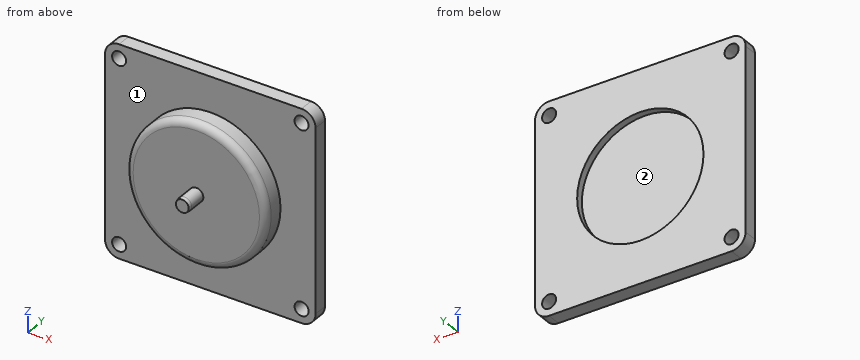
from build123d import *

# Parameters (mm, degrees)
SKETCH1_W           = 30
SKETCH1_H           = 30
BOSS_EXTRUDE1_DEPTH = 2
SKETCH2_R           = 9
CUT_EXTRUDE1_DEPTH  = 1
SKETCH3_R           = 10
BOSS_EXTRUDE2_DEPTH = 3
SKETCH4_R           = 1
BOSS_EXTRUDE3_DEPTH = 3
FILLET1_R           = 1
CHAMFER2_SIZE       = 0.5
CHAMFER2_SIZE2      = 0.08816349
SKETCH5_R           = 1
CUT_EXTRUDE2_DEPTH  = 3
FILLET2_R           = 2


with BuildPart() as part:
    # Sketch1 → Boss-Extrude1 (new body)
    with BuildSketch(Plane(origin=(0, 0, 0), x_dir=(1, 0, 0), z_dir=(0, 1, 0))):
        Rectangle(SKETCH1_W, SKETCH1_H)
    extrude(amount=BOSS_EXTRUDE1_DEPTH)

    # Sketch2 → Cut-Extrude1 (cut)
    with BuildSketch(Plane(origin=(0, 2, 0), x_dir=(1, 0, 0), z_dir=(0, 1, 0))):
        Circle(SKETCH2_R)
    extrude(amount=-CUT_EXTRUDE1_DEPTH, mode=Mode.SUBTRACT)

    # Sketch3 → Boss-Extrude2 (add)
    with BuildSketch(Plane.XZ):
        Circle(SKETCH3_R)
    extrude(amount=BOSS_EXTRUDE2_DEPTH)

    # Sketch4 → Boss-Extrude3 (add)
    with BuildSketch(Plane.XZ.offset(3)):
        Circle(SKETCH4_R)
    extrude(amount=BOSS_EXTRUDE3_DEPTH)

    # Fillet1
    fillet1_edges = [part.edges().sort_by_distance(p)[0] for p in [
        (-10, -3, 0),
    ]]
    fillet(fillet1_edges, radius=FILLET1_R)

    # Chamfer2
    chamfer2_edges = [part.edges().sort_by_distance(p)[0] for p in [
        (-1, -6, 0),
    ]]
    chamfer2_side = [part.faces().sort_by_distance(p)[0] for p in [
        (-1, -4.5, 0),
    ]]
    chamfer(chamfer2_edges, length=CHAMFER2_SIZE, length2=CHAMFER2_SIZE2, reference=chamfer2_side[0])

    # Sketch5 → Cut-Extrude2 (cut, through all)
    with BuildSketch(Plane.XZ):
        with Locations((-13, 13)):
            Circle(SKETCH5_R)
        with Locations((13, 13)):
            Circle(SKETCH5_R)
        with Locations((13, -13)):
            Circle(SKETCH5_R)
        with Locations((-13, -13)):
            Circle(SKETCH5_R)
    extrude(amount=-CUT_EXTRUDE2_DEPTH, mode=Mode.SUBTRACT)

    # Fillet2
    fillet2_edges = [part.edges().sort_by_distance(p)[0] for p in [
        (15, 1, 15),
        (-15, 1, 15),
        (-15, 1, -15),
        (15, 1, -15),
    ]]
    fillet(fillet2_edges, radius=FILLET2_R)


solid = part.part
Design review of the part built by this model. Coordinates are the model's own, in mm. Face numbers are marked on the shaded views. Give positions to 0.01 mm unless a question says otherwise; leave off trailing zeros. Loops run counter-clockwise (first coordinate to the right, second up) from the corner with the lowest first, then second, coordinate; pieces in that order, holes last. Notation, with made-up numbers: M -37.5,38.25 L 8.5,38.25 A19 cw 8.5,44.25 Z; hole C 77,6 d3. An arc over 180 degrees is marked long. Answer as a JSON object with one key per item and string values.
Item 1: We need section A-A (x = 0). State the section outline as (y, z) points.
Output values:
{"outline": "M -6,-0.91 L -5.5,-1 L -3,-1 L -3,-9 A1 ccw -2,-10 L 0,-10 L 0,-15 L 2,-15 L 2,-9 L 1,-9 L 1,9 L 2,9 L 2,15 L 0,15 L 0,10 L -2,10 A1 ccw -3,9 L -3,1 L -5.5,1 L -6,0.91 Z"}
Item 2: We need section B-B (y = -3.75). State the section outline as (x, z) points, and give its area (3 significant figures).
Output values:
{"outline": "C 0,0 d2", "area": "3.14 mm2"}
Item 3: Mouldability with a two-part tool opening along X and no side actions: class the marked faces 1 and 2 as pulls with the +X half, pulls with the -X half, needs draft (parallel to the pull), parting line crosses it, or undercut.
Output values:
{"face 1": "needs draft", "face 2": "undercut"}
Item 4: Wall thickness on line 1 along Z through (x, y) = (13, 0.6); line 2 along Z through (x, y) = (0, 1.25): over which ranges is each line inside the solid? List them lowest first.
Output values:
{"line 1": "z = -15 to -14, -12 to 12, 14 to 15", "line 2": "z = -15 to -9, 9 to 15"}
Item 5: For P1, Ø1, axis at x = -7.5, z = -0.5, coming from the +Y side; P2, Ø14.5, axis at x = 2, z = -1, coming from the -Y side; P3, Ø5, axis at x = -0.5, z = -10, coming from the -Y side, all flat-tipped, find the tip position at first contact; note any pin that passes through.
Output values:
{"P1": "stops at y = 1", "P2": "stops at y = -6", "P3": "stops at y = -3"}
